Geometry: final body of the model. Coordinates: model frame, mm. A direction names the side the tool comes from. Coordinates: 2 decimals unless noted, no trailing zeros. Write each loop counter-clockwise with the first axis right and the second up, starting at its lowest first coordinate (ties: lowest second). Pieces come first, ordered by that corner, then holes.
from build123d import *

# Parameters (mm, degrees)
F0_R      = 8.5
F1_DEPTH  = 13
F2_R      = 2.75
F3_DEPTH  = 13.001
F4_R      = 4.5
F5_DEPTH  = 10
F6_SIZE   = 0.2
F7_R      = 7.75
F7_R_2    = 5.25
F8_DEPTH  = 0.8
F9_DEPTH  = 1
F10_R     = 5.6
F10_R_2   = 4.5
F11_DEPTH = 1.5
F11_TAPER = 15


# Not quite as in the source:
# - a fillet or chamfer that OpenCascade refuses, or shapes differently, is made with other operations: its cross-section is extruded or revolved along the edge and cut away or added
# - a feature names something its author has since deleted; it is built from what else it names


with BuildPart() as f1:
    # F0 (on Top) → F1 (new body)
    with BuildSketch(Plane.XY):
        Circle(F0_R)
    extrude(amount=F1_DEPTH)

    # F2 (on face) → F3 (cut, through all)
    with BuildSketch(Plane.XY.offset(13)):
        Circle(F2_R)
    extrude(amount=-F3_DEPTH, mode=Mode.SUBTRACT)

    # F4 (on face) → F5 (cut)
    with BuildSketch(Plane.XY.offset(13)):
        Circle(F4_R)
    extrude(amount=-F5_DEPTH, mode=Mode.SUBTRACT)

    # F6
    f6_edges = [f1.edges().sort_by_distance(p)[0] for p in [
        (-8.5, 0, 13),
    ]]
    chamfer(f6_edges, length=F6_SIZE)

    # F7 (on face) → F8 (cut)
    with BuildSketch(Plane.XY.offset(13)):
        Circle(F7_R)
        Circle(F7_R_2, mode=Mode.SUBTRACT)
    extrude(amount=-F8_DEPTH, mode=Mode.SUBTRACT)

    # F9 (add): a face of the model
    f9_faces = [f1.faces().sort_by_distance(p)[0] for p in [
        (-5.101507576, 0, 13),
    ]]
    extrude(f9_faces, amount=F9_DEPTH)

    # F10 (on face) → F11 (join)
    with BuildSketch(Plane.XY.offset(14)):
        Circle(F10_R)
        Circle(F10_R_2, mode=Mode.SUBTRACT)
    extrude(amount=-F11_DEPTH, taper=F11_TAPER)

    # F12: chamfer of 0.5 on 2 edges, made by hand

    # F12_s1 → F12_t2 (revolve)
    with BuildSketch(Plane.XZ):
        Polygon((7.75, 12.7), (7.25, 12.2), (7.75, 12.2), align=None)
    revolve(axis=Axis((0, 0, 12.2), (0, 0, 1)))

    # F12_s3 → F12_t4 (revolve)
    with BuildSketch(Plane.XZ):
        Polygon((5.75, 12.2), (5.25, 12.7), (5.25, 12.2), align=None)
    revolve(axis=Axis((0, 0, 12.2), (0, 0, 1)))


solid = f1.part
Item 1: Pull-direction query (X, two-part tool) for faces 3 (the flat face through (4, 0, 0)), 4 (the flat face through (-4.9, 3.3, 12.2)), 5 (the cylindrical face through (4.57, 7.167, 6.31)); classes: released by +X, released by -X, zero draft, split by the parting line, or undercut.
Derived:
face 3: zero draft
face 4: undercut
face 5: split by the parting line
Item 2: Section A-A, the plane z = 4. Output: boundary loops of the cut face in (x, y), plus the area to 3 significant figures.
Derived:
outline: circle Ø17 at (0, 0); hole circle Ø9 at (0, 0)
area: 163 mm2
Item 3: Set-up query: faces 1 (the flat face through (0, 5, 14)), 2 (the cylindrical face through (-0.59, 4.46, 8.42)). Return all of +Z, -Z, +X, -X, +Y, -Y with unobstructed straight access to the full face (end or side cutting, diameter ignored); none if empty.
Derived:
face 1: +Z, +X, -X, +Y, -Y
face 2: +Z
Item 4: Material intervals for probe 1 along Y at (x, z) = (0, 12.95); probe 2 along Y at (x, z) = (0, 6); probe 3 along Z at (x, y) = (6, 0.25), sorted ascending.
Derived:
probe 1: y = -8.35 to -7.75, -5.32 to -4.5, 4.5 to 5.32, 7.75 to 8.35
probe 2: y = -8.5 to -4.5, 4.5 to 8.5
probe 3: z = 0 to 12.2
Item 5: Pin query (flat end, axial travel): pin 1 (3 mm diameter, centred on x = 3, z = 8.5, fed in from -Y); pin 2 (10 mm diameter, centred on x = 4.5, y = 5.5, fed in from +Z); pin 3 (5 mm diameter, centred on x = 6.5, z = 7, fed in from +Y); pin 4 (4.5 mm diameter, centred on x = 1.5, y = -1, fed in from +Z). Return the tip coordinate at first contact, or that it passes through.
Derived:
pin 1: stops at y = -8.37
pin 2: stops at z = 14
pin 3: stops at y = 7.5
pin 4: stops at z = 3
Item 6: Section B-B, the plane x = 0. Output: boundary loops of the cut face in (y, z).
Derived:
outline: (-8.5, 0) - (-2.75, 0) - (-2.75, 3) - (-4.5, 3) - (-4.5, 14) - (-5.6, 14) - (-5.25, 12.7) - (-5.75, 12.2) - (-7.25, 12.2) - (-7.75, 12.7) - (-7.75, 13) - (-8.3, 13) - (-8.5, 12.8) - close; (2.75, 0) - (8.5, 0) - (8.5, 12.8) - (8.3, 13) - (7.75, 13) - (7.75, 12.7) - (7.25, 12.2) - (5.75, 12.2) - (5.25, 12.7) - (5.6, 14) - (4.5, 14) - (4.5, 3) - (2.75, 3) - close
